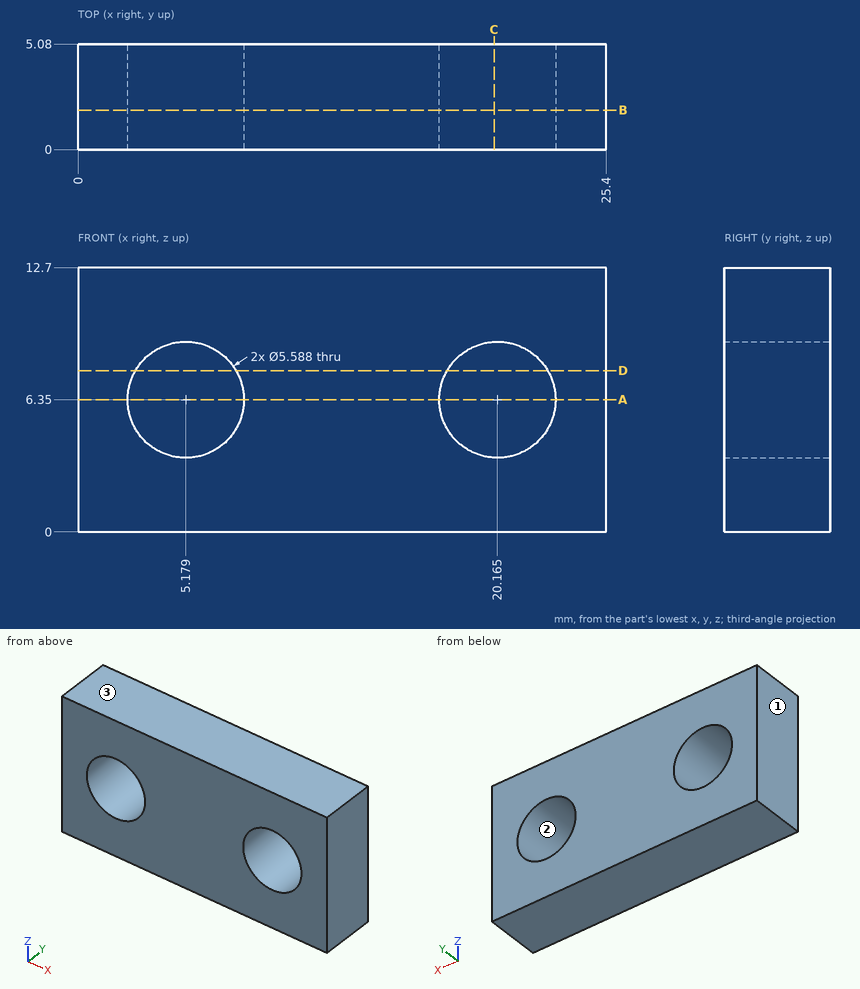
Design review of the part shown in the three views and the two pictorial views. Dimensions are in mm from the part's minimum x, y and z. Round coordinates to 2 decimals unless told otherwise and drop trailing zeros. Order: outer loops, then holes, each group sorted by start corner. A loop starts at its lowest first (then second) coordinate and runs counter-clockwise, first axis right, second up. Notation, with made-up numbers: (44, 43) -> (51, 43) arc R13 ccw to (51, 60) -> close; hole circle Ø10 at (77, -19.5). An arc over 180 degrees is marked (long way). Write item = value, one per line. Start each with the question number.
1) Take a section at D-D on z = 7.75. State the section outline as (x, y) points.
2) Take a section at B-B on y = 1.9. Count the separate pieces of the cut face and the enclosed holes in it.
3) Take a section at C-C on x = 20. State the section outline as (y, z) points, plus the area to 3 significant figures.
4) Take a section at A-A on z = 6.35. State the section outline as (x, y) points (1 decimal).
5) To check wall thickness, follow line 1 (X direction, y = 3.4, z = 6.35) (1 decimal); line 2 (Z direction, x = 5, y = 3.45); line 3 (X direction, y = 3.75, z = 5.5). State the ranges of each line that lie inside material, in increasing order. Write a range as from..to.
6) Insertion check: pin 1 (1.5 mm diameter, centred on x = 19.5, z = 8, fed in from -Y). The pin has a flat end and moves straight along its axis. Give the tip position at first contact, or say it passes through.
7) The part is to be moulded in two halves that separate along X. For the marked faces 1, 2 and 3, say which applies: +X half, -X half, draft (parallel to the pull), parting line (faces both ways), or undercut.
Verdict:
q1.outline = (0, 0) -> (2.76, 0) -> (2.76, 5.08) -> (0, 5.08) -> close; (7.6, 0) -> (17.75, 0) -> (17.75, 5.08) -> (7.6, 5.08) -> close; (22.58, 0) -> (25.4, 0) -> (25.4, 5.08) -> (22.58, 5.08) -> close
q2.separate_pieces = 1
q2.enclosed_holes = 2
q3.outline = (0, 0) -> (5.08, 0) -> (5.08, 3.56) -> (0, 3.56) -> close; (0, 9.14) -> (5.08, 9.14) -> (5.08, 12.7) -> (0, 12.7) -> close
q3.area = 36.2 mm2
q4.outline = (0, 0) -> (2.4, 0) -> (2.4, 5.1) -> (0, 5.1) -> close; (8, 0) -> (17.4, 0) -> (17.4, 5.1) -> (8, 5.1) -> close; (23, 0) -> (25.4, 0) -> (25.4, 5.1) -> (23, 5.1) -> close
q5.line_1 = 0..2.4, 8..17.4, 23..25.4
q5.line_2 = 0..3.56, 9.14..12.7
q5.line_3 = 0..2.52, 7.84..17.5, 22.83..25.4
q6.pin_1 = through
q7.face_1 = -X half
q7.face_2 = undercut
q7.face_3 = draft
